```python
from build123d import *

# Parameters (mm, degrees)
SKETCH1_W           = 5
SKETCH1_H           = 15
BOSS_EXTRUDE1_DEPTH = 4
SKETCH2_W           = 11
SKETCH2_H           = 21
BOSS_EXTRUDE2_DEPTH = 2
FILLET1_R           = 0.5
FILLET2_R           = 1.5


with BuildPart() as part:
    # Sketch1 → Boss-Extrude1 (new body)
    with BuildSketch(Plane(origin=(0, 0, 0), x_dir=(1, 0, 0), z_dir=(0, 1, 0))):
        with Locations((3, 8)):
            Rectangle(SKETCH1_W, SKETCH1_H)
    extrude(amount=BOSS_EXTRUDE1_DEPTH)

    # Sketch2 → Boss-Extrude2 (add)
    with BuildSketch(Plane.XZ):
        with Locations((3, -8)):
            Rectangle(SKETCH2_W, SKETCH2_H)
    extrude(amount=BOSS_EXTRUDE2_DEPTH)

    # Fillet1
    fillet1_edges = [part.edges().sort_by_distance(p)[0] for p in [
        (5.5, 4, -8),
        (3, 4, -15.5),
        (0.5, 4, -8),
        (0.5, 2, -15.5),
        (5.5, 2, -15.5),
        (5.5, 2, -0.5),
        (0.5, 2, -0.5),
        (3, 4, -0.5),
    ]]
    fillet(fillet1_edges, radius=FILLET1_R)

    # Fillet2
    fillet2_edges = [part.edges().sort_by_distance(p)[0] for p in [
        (8.5, -1, -18.5),
        (8.5, -1, 2.5),
        (-2.5, -1, 2.5),
        (-2.5, -1, -18.5),
        (8.5, -2, -8),
        (3, -2, 2.5),
        (-2.5, -2, -8),
        (3, -2, -18.5),
    ]]
    fillet(fillet2_edges, radius=FILLET2_R)


solid = part.part
```
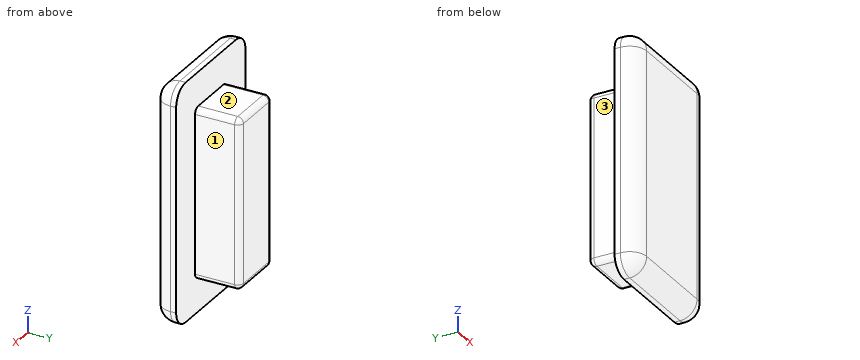
Could you check a few things on this model? Use its own coordinates, in mm. Face numbers are marked on the shaded views. A direction names the side the tool comes from. Round coordinates to 2 decimals unless told otherwise and drop trailing zeros. Loops run counter-clockwise (first coordinate to the right, second up) from the corner with the lowest first, then second, coordinate; pieces in that order, holes last.
Q1. Please list where these lines run through material, in increasing order: L1, parallel to X at y = 1.9, z = -5.5; L2, parallel to Z at x = 4, y = 3.1; L3, parallel to Y at x = 5.75, z = -4.
Q2. I want a section at B-B (x = 5.75). Write out the boundary of the cut face in (y, z).
Q3. I want a section at D-D (x = 3.5). Write out the boundary of the cut face in (y, z), and give its area (3 significant figures).
Q4. I want a section at A-A (y = 2.4). Write out the boundary of the cut face in (x, z), and give its area (3 significant figures).
Q5. For P1, Ø1, axis at y = 1, z = -6.5, coming from the +X side; P2, Ø1, axis at x = 2, y = 3, coming from the +Z side; P3, Ø1.8, axis at x = 2.5, y = 2, coming from the -Z side, each with a flat end and sliding along its axis, tell me the tip position at first contact or that it passes through.
Q6. I want a section at C-C (z = -5.5). Write out the boundary of the cut face in (x, y), and give its area (3 significant figures).
Q7. On a 3-axis mill with a long thin cutter (end or side, diameter ignored), from which of +Z, -Z, +X, -X, +Y, -Y can I reach the whole of each face in a straight line? I mean the marked faces 1, 2 and 3. Say none if no direction works.
Answer below:
1. L1: x = 0.5 to 5.5
1. L2: z = -15.5 to -0.5
1. L3: y = -2 to 0
2. outline: (-2, -17) arc R1.5 ccw to (-0.5, -18.5) - (0, -18.5) - (0, 2.5) - (-0.5, 2.5) arc R1.5 ccw to (-2, 1) - close
3. outline: (-2, -17) arc R1.5 ccw to (-0.5, -18.5) - (0, -18.5) - (0, -15.5) - (3.5, -15.5) arc R0.5 ccw to (4, -15) - (4, -1) arc R0.5 ccw to (3.5, -0.5) - (0, -0.5) - (0, 2.5) - (-0.5, 2.5) arc R1.5 ccw to (-2, 1) - close
3. area: 101 mm2
4. outline: (0.5, -15) arc R0.5 ccw to (1, -15.5) - (5, -15.5) arc R0.5 ccw to (5.5, -15) - (5.5, -1) arc R0.5 ccw to (5, -0.5) - (1, -0.5) arc R0.5 ccw to (0.5, -1) - close
4. area: 74.8 mm2
5. P1: stops at x = 5.5
5. P2: stops at z = -0.5
5. P3: stops at z = -15.5
6. outline: (-2.5, -0.5) arc R1.5 ccw to (-1, -2) - (7, -2) arc R1.5 ccw to (8.5, -0.5) - (8.5, 0) - (5.5, 0) - (5.5, 3.5) arc R0.5 ccw to (5, 4) - (1, 4) arc R0.5 ccw to (0.5, 3.5) - (0.5, 0) - (-2.5, 0) - close
6. area: 40.9 mm2
7. face 1: +Z, -Z, +X, +Y
7. face 2: +Z, +X, -X, +Y
7. face 3: +Z, -Z, -X, +Y
